Input: part model. Units: mm. Frame: model coordinates. Face numbers are marked on the shaded views. A direction names the side the tool comes from. Give positions to 0.01 mm unless a question says otherwise; leave off trailing zeros. Order: outer loops, then holes, each group sorted by start corner. A loop starts at its lowest first (then second) coordinate and runs counter-clockwise, first axis right, second up. Notation, with made-up numbers: M -33,-21.75 L -18,-21.75 A19 ccw -18,15.25 Z; hole C 1,26.25 d4. An arc over 180 degrees is marked long. Use a Markdown table: item, result.
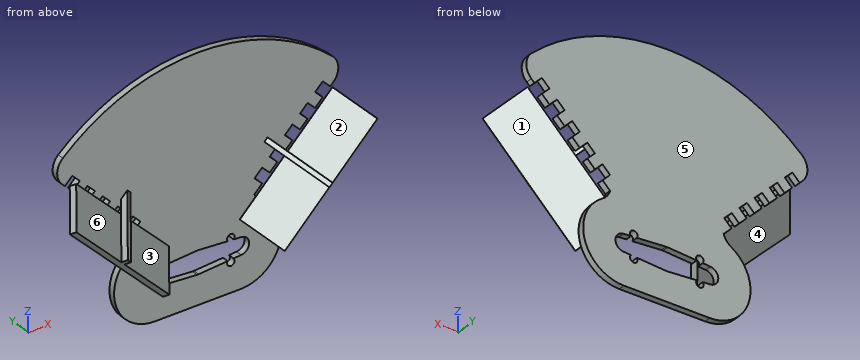
from build123d import *

# Parameters (mm, degrees)
SKETCH_1_W          = 180
SKETCH_1_H          = 123.475609756
EXTRUDE_1_DEPTH     = 3
SKETCH_2_OUTSIDE_W  = 225.66
SKETCH_2_OUTSIDE_H  = 169.136
CUT_EXTRUDE_1_DEPTH = 10
EXTRUDE_3_DEPTH     = 1.5
EXTRUDE_4_DEPTH     = 3
CUT_EXTRUDE_2_DEPTH = 13
EXTRUDE_5_DEPTH     = 3
CUT_EXTRUDE_4_DEPTH = 5


with BuildPart() as part:
    # 草图1 → 凸台-拉伸1 (new body)
    with BuildSketch(Plane(origin=(0, 0, 0), x_dir=(1, 0, 0), z_dir=(0, 1, 0))):
        Rectangle(SKETCH_1_W, SKETCH_1_H)
    extrude(amount=EXTRUDE_1_DEPTH)

    # 草图2 outside → 切除-拉伸1 (cut)
    with BuildSketch(Plane(origin=(0, 3, 0), x_dir=(1, 0, 0), z_dir=(0, 1, 0))):
        Rectangle(SKETCH_2_OUTSIDE_W, SKETCH_2_OUTSIDE_H)
        with BuildLine():
            Line((63.393156076, -4.57196386), (17.660793085, 41.160399131))
            ThreePointArc((17.660793085, 41.160399131), (13.212332654, 43.192679399), (8.519172912, 41.81673793))
            ThreePointArc((8.519172912, 41.81673793), (0.135427504, 39.028910463), (-8.248317905, 41.81673793))
            ThreePointArc((-8.248317905, 41.81673793), (-12.941477647, 43.192679399), (-17.389938078, 41.160399131))
            Line((-17.389938078, 41.160399131), (-63.122301068, -4.57196386))
            ThreePointArc((-63.122301068, -4.57196386), (-65.463259353, -10.415886745), (-62.851632161, -16.14396878))
            ThreePointArc((-62.851632161, -16.14396878), (0.135427504, -40.524587109), (63.122487168, -16.14396878))
            ThreePointArc((63.122487168, -16.14396878), (65.73411436, -10.415886745), (63.393156076, -4.57196386))
        make_face(mode=Mode.SUBTRACT)
    extrude(amount=-CUT_EXTRUDE_1_DEPTH, mode=Mode.SUBTRACT)

    # 草图4 → 凸台-拉伸3 (add, symmetric)
    with BuildSketch(Plane(origin=(11.169764148, 15.796431947, -11.169764148), x_dir=(-0.8660254037844386, 0.40824829046386313, -0.288675134594813), z_dir=(-0.5000000000000001, -0.7071067811865476, 0.49999999999999983))):
        Polygon((-42.887555568, 35.134950382), (-23.8863598, 8.357630936), (-25.587706579, 7.150354633), (-44.588902348, 33.927674079), align=None)
    extrude_3 = extrude(amount=EXTRUDE_3_DEPTH, both=True)

    # 草图5 → 凸台-拉伸4 (add)
    with BuildSketch(Plane(origin=(11.919764148, 16.857092119, -11.919764148), x_dir=(0.8660254037844387, -0.408248290463863, 0.2886751345948128), z_dir=(0.49999999999999994, 0.7071067811865477, -0.4999999999999999))):
        Polygon((5.305528324, 33.262652537), (23.440849678, 58.85571886), (73.424034658, 23.437488372), (55.288713303, -2.155577951), align=None)
    extrude_4 = extrude(amount=EXTRUDE_4_DEPTH)

    # 草图6 → 切除-拉伸2 (cut)
    with BuildSketch(Plane(origin=(13.419764148, 18.978412462, -13.419764148), x_dir=(0.8660254037844387, -0.40824829046386313, 0.2886751345948128), z_dir=(0.5, 0.7071067811865477, -0.49999999999999983))):
        Polygon((17.332913893, 50.236031202), (67.316098873, 14.817800715), (73.424034658, 23.437488372), (23.440849678, 58.85571886), align=None)
    cut_extrude_2 = extrude(amount=-CUT_EXTRUDE_2_DEPTH, mode=Mode.SUBTRACT)

    # 镜向2: 凸台-拉伸3, 凸台-拉伸4, 切除-拉伸2 across plane
    add(extrude_3.mirror(Plane(origin=(0, 0, 0), x_dir=(0, 0, 1), z_dir=(1, 0, 0))))
    add(extrude_4.mirror(Plane(origin=(0, 0, 0), x_dir=(0, 0, 1), z_dir=(1, 0, 0))))
    add(cut_extrude_2.mirror(Plane(origin=(0, 0, 0), x_dir=(0, 0, 1), z_dir=(1, 0, 0))), mode=Mode.SUBTRACT)

    # 草图7 → 凸台-拉伸5 (add)
    with BuildSketch(Plane(origin=(0, 3, 0), x_dir=(1, 0, 0), z_dir=(0, 1, 0))):
        with BuildLine():
            Line((-19.864572496, 72.089252639), (20.135427504, 72.089252639))
            ThreePointArc((20.135427504, 72.089252639), (38.479418015, 58.205265935), (30.099048805, 36.780129142))
            ThreePointArc((30.099048805, 36.780129142), (26.400179556, 30.999210524), (28.649163581, 24.515174385))
            Line((28.649163581, 24.515174385), (-28.378308574, 24.515174385))
            ThreePointArc((-28.378308574, 24.515174385), (-26.129324549, 30.999210524), (-29.828193798, 36.780129142))
            ThreePointArc((-29.828193798, 36.780129142), (-38.208563008, 58.205265935), (-19.864572496, 72.089252639))
        make_face()
        with BuildLine():
            Line((20.415427504, 57.019098429), (16.875331791, 57.267514495))
            ThreePointArc((16.875331791, 57.267514495), (15.677130379, 60.161371451), (14.08652518, 57.463211003))
            Line((14.08652518, 57.463211003), (0.513427504, 58.415664216))
            ThreePointArc((0.513427504, 58.415664216), (0.135427504, 58.428910463), (-0.242572496, 58.415664216))
            Line((-0.242572496, 58.415664216), (-13.815670173, 57.463211003))
            ThreePointArc((-13.815670173, 57.463211003), (-15.406275372, 60.161371451), (-16.604476783, 57.267514495))
            Line((-16.604476783, 57.267514495), (-20.144572496, 57.019098429))
            ThreePointArc((-20.144572496, 57.019098429), (-23.864572496, 53.028910463), (-20.144572496, 49.038722498))
            Line((-20.144572496, 49.038722498), (-16.604476783, 48.790306431))
            ThreePointArc((-16.604476783, 48.790306431), (-15.406275372, 45.896449475), (-13.815670173, 48.594609923))
            Line((-13.815670173, 48.594609923), (-0.242572496, 47.64215671))
            ThreePointArc((-0.242572496, 47.64215671), (0.135427504, 47.628910463), (0.513427504, 47.64215671))
            Line((0.513427504, 47.64215671), (14.08652518, 48.594609923))
            ThreePointArc((14.08652518, 48.594609923), (15.677130379, 45.896449475), (16.875331791, 48.790306431))
            Line((16.875331791, 48.790306431), (20.415427504, 49.038722498))
            ThreePointArc((20.415427504, 49.038722498), (24.135427504, 53.028910463), (20.415427504, 57.019098429))
        make_face(mode=Mode.SUBTRACT)
    extrude(amount=-EXTRUDE_5_DEPTH)

    # 草图8 → 切除-拉伸4 (cut)
    with BuildSketch(Plane(origin=(0, 3, 0), x_dir=(1, 0, 0), z_dir=(0, 1, 0))):
        Polygon((54.918650137, -3.168525733), (58.454184043, -6.704059639), (61.989717949, -3.168525733), (58.454184043, 0.367008173), align=None)
        Polygon((51.383116231, 7.438075985), (47.847582325, 3.902542079), (51.383116231, 0.367008173), (54.918650137, 3.902542079), align=None)
        Polygon((44.31204842, 14.509143797), (40.776514514, 10.973609891), (44.31204842, 7.438075985), (47.847582325, 10.973609891), align=None)
        Polygon((37.240980608, 21.580211608), (33.705446702, 18.044677703), (37.240980608, 14.509143797), (40.776514514, 18.044677703), align=None)
        Polygon((30.169912796, 28.65127942), (26.63437889, 25.115745514), (30.169912796, 21.580211608), (33.705446702, 25.115745514), align=None)
        Polygon((-33.705446702, 25.115745514), (-30.169912796, 28.65127942), (-26.63437889, 25.115745514), (-30.169912796, 21.580211608), align=None)
        Polygon((-40.776514514, 18.044677703), (-37.240980608, 21.580211608), (-33.705446702, 18.044677703), (-37.240980608, 14.509143797), align=None)
        Polygon((-47.847582325, 10.973609891), (-44.31204842, 14.509143797), (-40.776514514, 10.973609891), (-44.31204842, 7.438075985), align=None)
        Polygon((-54.918650137, 3.902542079), (-51.383116231, 7.438075985), (-47.847582325, 3.902542079), (-51.383116231, 0.367008173), align=None)
        Polygon((-58.454184043, 0.367008173), (-54.918650137, -3.168525733), (-58.454184043, -6.704059639), (-61.989717949, -3.168525733), align=None)
    extrude(amount=-CUT_EXTRUDE_4_DEPTH, mode=Mode.SUBTRACT)


solid = part.part
1) Cut plane A-A on z = -34.5. Return loops of the section in (x, y), and give its area (3 significant figures).
Response values:
| item | result |
|---|---|
| outline | M -43.34,-17.09 L -40.35,-19.21 L -19.56,-4.51 L -22.56,-2.39 Z; M -27.44,0 L 27.71,0 L 27.71,3 L -27.44,3 Z; M 19.56,-4.51 L 40.35,-19.21 L 43.34,-17.09 L 22.56,-2.39 Z |
| area | 342 mm² |
2) Cut plane D-D on x = -11. Return loops of the section in (y, z), and give its area (3 significant figures).
Response values:
| item | result |
|---|---|
| outline | M 0,-72.09 L 3,-72.09 L 3,-57.66 L 0,-57.66 Z; M 0,-48.4 L 3,-48.4 L 3,39.86 L 0,39.86 Z |
| area | 308 mm² |
3) Cut plane C-C on y = -10. Return loops of the section in (x, z), and give its area (3 significant figures).
Response values:
| item | result |
|---|---|
| outline | M -66.72,-1.1 L -23.4,-44.42 L -20.4,-41.42 L -41.31,-20.51 L -38.31,-17.51 L -39.78,-16.04 L -42.78,-19.04 L -63.72,1.9 Z; M 20.4,-41.42 L 23.4,-44.42 L 66.72,-1.1 L 63.72,1.9 L 42.78,-19.04 L 39.78,-16.04 L 38.31,-17.51 L 41.31,-20.51 Z |
| area | 538 mm² |
4) Reachability of the marked faces 1, 2 and 3 from +Z, -Z, +X, -X, +Y, -Y: full face, straight path, thin tool, end or side. Return the list, or none.
Response values:
| item | result |
|---|---|
| face 1 | -Z, +X |
| face 2 | +Z, -Y |
| face 3 | -Y |
5) Cut plane B-B on x = -56.5. Return loops of the section in (y, z), and give its area (3 significant figures).
Response values:
| item | result |
|---|---|
| outline | M -19.19,-18.32 L -17.07,-21.32 L -2.35,-0.51 L -4.47,2.49 Z; M 0,-2.05 L 3,-2.05 L 3,1.59 L 0,1.59 Z; M 0,4.75 L 3,4.75 L 3,21.43 L 0,21.43 Z |
| area | 149 mm² |
6) First-contact query: pin 1 Ø10 at (x, z) = (3.5, -27) entering from -Y; pin 2 Ø3 at (x, z) = (15.55, -58.42) entering from +Y; pin 3 Ø3 at (y, z) = (-11, -10) entering from -X; pin 4 Ø8 at (x, z) = (28, -32.5) entering from +Y. Flat tips, straight axial feed; report the tip coordinate or a pass-through.
Response values:
| item | result |
|---|---|
| pin 1 | stops at y = 0 |
| pin 2 | passes through |
| pin 3 | stops at x = -61.83 |
| pin 4 | stops at y = 3 |
7) Mould query, pull axis X, two halves, no side actions, for the marked faces 4, 5 and 6. Classes: released by +X, released by -X, zero draft, split by the parting line, or undercut.
Response values:
| item | result |
|---|---|
| face 4 | released by -X |
| face 5 | zero draft |
| face 6 | undercut |
8) Material intervals for line 1 (Y direction, x = -26, z = 33.5); line 2 (X direction, y = -10.75, z = -32); line 3 (X direction, y = -6.5, z = -3), sorted ascending. Write a range as from..to.
Response values:
| item | result |
|---|---|
| line 1 | y = 0..3 |
| line 2 | x = -36.88..-30.88, 30.88..36.88 |
| line 3 | x = -59.87..-53.87, 53.87..59.87 |
